Input: part model. Units: mm. Frame: model coordinates. Round coordinates to 2 decimals unless told otherwise and drop trailing zeros. Loops run counter-clockwise (first coordinate to the right, second up) from the corner with the lowest first, then second, coordinate; pieces in that order, holes last. Notation, with made-up numbers: (80.5, -19.5) -> (125.5, -19.5) arc R33 cw to (125.5, 9.5) -> close; hole circle Ø2 at (26.5, -2.5). An arc over 180 degrees is marked (long way). One line per question, with ' | ' between items. Start each with the question number.
Q1. Material intervals for L1, parallel to Y at x = 0, z = 9; L2, parallel to Z at x = -2.6, y = 1.15, sorted ascending.
Q2. Contact query for flat-ended pins moving along their axis: P1, Ø1.5, axis at x = -1.5, z = 7, coming from the +Y side; P2, Ø1, axis at x = 1, y = -2, coming from the +Z side; P3, Ø1.5, axis at x = 1.5, z = 16, coming from the -Y side. Output: stop coordinate, or through.
Q3. Mould query, pull axis Y, two halves, no side actions, for faces 1 (the face through (-1.4, 0.06, 8.87)), 2 (the face through (0, 0, 18)). Classes: pulls with the +Y half, pulls with the -Y half, needs draft (parallel to the pull), parting line crosses it, or undercut.
Q4. Cut plane A-A on z = 8.25. Return loops of the section in (x, y).
from build123d import *

# Parameters (mm, degrees)
ESQUISSE1_R        = 1.4
BOSS_EXTRU_1_DEPTH = 18
ESQUISSE2_R        = 3
BOSS_EXTRU_2_DEPTH = 2
CONG_2_R           = 2


with BuildPart() as part:
    # Esquisse1 → Boss.-Extru.1 (new body)
    with BuildSketch(Plane.XY):
        Circle(ESQUISSE1_R)
    extrude(amount=BOSS_EXTRU_1_DEPTH)

    # Esquisse2 → Boss.-Extru.2 (add)
    with BuildSketch(Plane(origin=(0, 0, 0), x_dir=(-1, 0, 0), z_dir=(0, 0, -1))):
        Circle(ESQUISSE2_R)
    extrude(amount=BOSS_EXTRU_2_DEPTH)

    # Congé2
    cong_2_edges = [part.edges().sort_by_distance(p)[0] for p in [
        (3, 0, -2),
    ]]
    fillet(cong_2_edges, radius=CONG_2_R - 0.0001)  # a hair under: the kernel refuses the full size


solid = part.part
Results:
1) L1: -1.4 to 1.4 | L2: -0.78 to 0
2) P1: y = 1.18 | P2: z = 0 | P3: y = -1.18
3) face 1: parting line crosses it | face 2: needs draft
4) outline: circle Ø2.8 at (0, 0)
